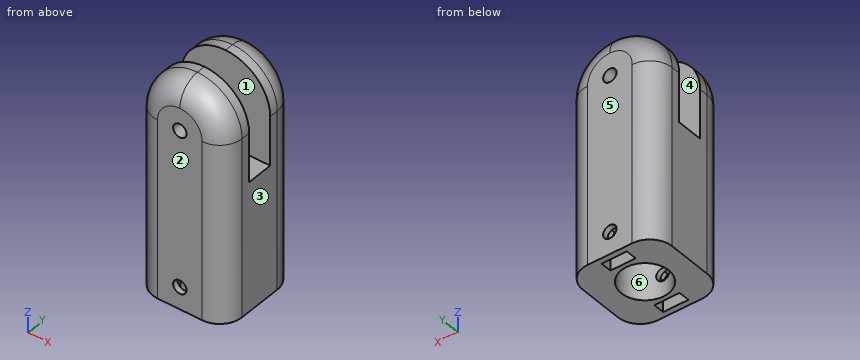
```python
from build123d import *

# Parameters (mm, degrees)
SKETCH1_W           = 20
SKETCH1_H           = 20
SKETCH1_R           = 5.3
BOSS_EXTRUDE1_DEPTH = 25
SKETCH2_W           = 20
SKETCH2_H           = 20
BOSS_EXTRUDE2_DEPTH = 25
SKETCH4_W           = 20
SKETCH4_H           = 6
CUT_EXTRUDE1_DEPTH  = 21
CUT_EXTRUDE2_REACH  = 59.446
SKETCH5_R           = 1.5
FILLET2_R           = 10
FILLET3_R           = 5
SKETCH6_W           = 5.65
SKETCH6_H           = 2.5
CUT_EXTRUDE3_DEPTH  = 8
CHAMFER1_SIZE       = 1


with BuildPart() as part:
    # Sketch1 → Boss-Extrude1 (new body)
    with BuildSketch(Plane.XY):
        with Locations((10, 10)):
            Rectangle(SKETCH1_W, SKETCH1_H)
        with Locations((10, 10)):
            Circle(SKETCH1_R, mode=Mode.SUBTRACT)
    extrude(amount=BOSS_EXTRUDE1_DEPTH)

    # Sketch2 → Boss-Extrude2 (add)
    with BuildSketch(Plane.XY.offset(25)):
        with Locations((10, 10)):
            Rectangle(SKETCH2_W, SKETCH2_H)
    extrude(amount=BOSS_EXTRUDE2_DEPTH)

    # Sketch4 → Cut-Extrude1 (cut)
    with BuildSketch(Plane.XY.offset(50)):
        with Locations((10, 10)):
            Rectangle(SKETCH4_W, SKETCH4_H)
    extrude(amount=-CUT_EXTRUDE1_DEPTH, mode=Mode.SUBTRACT)

    # Cut-Extrude2: up to this face of the body (flat: up to its plane)
    cut_extrude2_end = Plane(part.part.faces().sort_by_distance((10, 0, 25))[0])
    # Sketch5 → Cut-Extrude2 (cut, up to the picked face)
    with BuildSketch(Plane(origin=(0, 20, 0), x_dir=(1, 0, 0), z_dir=(0, 1, 0)), mode=Mode.PRIVATE) as cut_extrude2_sk1:
        with Locations(Location((10, -5, 0), (0, 0, 270))):
            Circle(SKETCH5_R)
    cut_extrude2_tool1 = split(extrude(cut_extrude2_sk1.sketch, amount=-CUT_EXTRUDE2_REACH, mode=Mode.PRIVATE), bisect_by=cut_extrude2_end, keep=Keep.BOTH, mode=Mode.PRIVATE)
    # Sketch5 → Cut-Extrude2 (cut, up to the picked face)
    with BuildSketch(Plane(origin=(0, 20, 0), x_dir=(1, 0, 0), z_dir=(0, 1, 0)), mode=Mode.PRIVATE) as cut_extrude2_sk2:
        with Locations(Location((10, -40, 0), (0, 0, 270))):
            Circle(SKETCH5_R)
    cut_extrude2_tool2 = split(extrude(cut_extrude2_sk2.sketch, amount=-CUT_EXTRUDE2_REACH, mode=Mode.PRIVATE), bisect_by=cut_extrude2_end, keep=Keep.BOTH, mode=Mode.PRIVATE)
    add(cut_extrude2_tool1.solids().sort_by(Axis((10, 20, 5), (0, -1, 0)))[0], mode=Mode.SUBTRACT)
    add(cut_extrude2_tool2.solids().sort_by(Axis((10, 20, 40), (0, -1, 0)))[0], mode=Mode.SUBTRACT)

    # Fillet2
    fillet2_edges = [part.edges().sort_by_distance(p)[0] for p in [
        (0, 16.5, 50),
        (0, 3.5, 50),
        (20, 3.5, 50),
        (20, 16.5, 50),
    ]]
    fillet(fillet2_edges, radius=FILLET2_R - 0.0001)  # a hair under: the kernel refuses the full size

    # Fillet3
    fillet3_edges = [part.edges().sort_by_distance(p)[0] for p in [
        (0, 20, 20.00005),
        (0, 0, 20.00005),
        (20, 20, 20.00005),
        (17.071097101, 20, 47.071097101),
        (2.928902899, 20, 47.071097101),
        (20, 0, 20.00005),
        (17.071097101, 0, 47.071097101),
        (2.928902899, 0, 47.071097101),
    ]]
    fillet(fillet3_edges, radius=FILLET3_R)

    # Sketch6 → Cut-Extrude3 (cut)
    with BuildSketch(Plane(origin=(0, 0, 0), x_dir=(-1, 0, 0), z_dir=(0, 0, -1))):
        with Locations((-10, 17.5)):
            Rectangle(SKETCH6_W, SKETCH6_H)
        with Locations((-10, 2.5)):
            Rectangle(SKETCH6_W, SKETCH6_H)
    extrude(amount=-CUT_EXTRUDE3_DEPTH, mode=Mode.SUBTRACT)

    # Chamfer1
    chamfer1_edges = [part.edges().sort_by_distance(p)[0] for p in [
        (12.825, 17.5, 8),
        (7.175, 17.5, 8),
        (12.825, 2.5, 8),
        (7.175, 2.5, 8),
    ]]
    chamfer(chamfer1_edges, length=CHAMFER1_SIZE)


solid = part.part
```
Work out the finished part from the listing and answer in its coordinate system (mm). Face numbers are marked on the shaded views. A direction names the side the tool comes from. Give positions to 0.01 mm unless a question says otherwise; leave off trailing zeros. Order: outer loops, then holes, each group sorted by start corner. A loop starts at its lowest first (then second) coordinate and runs counter-clockwise, first axis right, second up. Notation, with made-up numbers: (80.25, -35) -> (129.25, -35) arc R15 ccw to (129.25, -9) -> close; hole circle Ø11 at (61, 27.5). An arc over 180 degrees is marked (long way). Answer as CSV lines item,"result". Start each with the question number.
(1) Section D-D, the plane y = 10 is taken. Write down the section's boundary in (x, z).
(2) Consider line 1 along Y through (x, z) = (12.5, 6.5); line 2 along Y through (x, z) = (8.5, 38.5); line 3 along X through (y, z) = (2, 3.5) (3 decimals). Determine where each line is inside the solid, lowest interval first.
(3) For a pull along Y with two mould halves and no side action, classify the marked faces 3, 4, 5 and 6 as released by +Y, released by -Y, zero draft, split by the parting line, or undercut.
(4) Which of the six approach directions +Z, -Z, +X, -X, +Y, -Y give full straight-line access (tool end or side, diameter ignored) to the marked faces 1 and 2?
(5) Section C-C, the plane z = 23 is taken. Write down the section's boundary in (x, y), plus the area to 3 significant figures.
(6) Each of these flat-tipped pins is pushed along its axis until it touches: pin 1 Ø2 at (y, z) = (2.5, 17) entering from +X; pin 2 Ø2 at (y, z) = (2, 4) entering from -X; pin 3 Ø1 at (y, z) = (17.5, 44) entering from +X. Where does it stop, or does it pass through?
Entries:
1,outline,"(0, 0) -> (4.7, 0) -> (4.7, 25) -> (15.3, 25) -> (15.3, 0) -> (20, 0) -> (20, 29) -> (0, 29) -> close"
2,line 1,"0 to 1.25, 3.75 to 5.33, 14.67 to 16.25, 18.75 to 20"
2,line 2,"0 to 7, 13 to 20"
2,line 3,"1 to 7.175, 12.825 to 19"
3,face 3,"zero draft"
3,face 4,"undercut"
3,face 5,"released by +Y"
3,face 6,"undercut"
4,face 1,"+Z, +X, -X"
4,face 2,"+Z, -Z, +X, -X, -Y"
5,outline,"(0, 5) arc R5 ccw to (5, 0) -> (15, 0) arc R5 ccw to (20, 5) -> (20, 15) arc R5 ccw to (15, 20) -> (5, 20) arc R5 ccw to (0, 15) -> close; hole circle Ø10.6 at (10, 10)"
5,area,"290 mm²"
6,pin 1,"x = 19.77"
6,pin 2,"x = 0.42"
6,pin 3,"x = 18.79"
